Can you work these out from the drawing? Everything is in mm from the part's minimum corner. A direction names the side the tool comes from. Give positions to 0.01 mm unless a question says otherwise; leave off trailing zeros. Order: outer loops, then holes, each group sorted by start corner. A loop starts at its lowest first (then second) coordinate and runs counter-clockwise, first axis right, second up. Notation, with made-up numbers: (-34.5, 58) -> (16.5, 58) arc R23 cw to (16.5, 72) -> close; hole circle Ø9 at (23, -36.75). An arc over 180 degrees is marked (long way). Answer as CSV lines item,"result". Start each with the question number.
(1) I want a section at B-B (z = 32.5). Please give me the cut outline in (x, y), plus the area to 3 significant figures.
(2) I want a section at D-D (y = 16). Please give me the cut outline in (x, z).
(3) I need wall thicknesses on L1, parallel to X at y = 59, z = 6; L2, parallel to X at y = 18, z = 8.5. Which ranges of each line are inside material? Lowest first, please.
(4) I want a section at C-C (y = 73). Please give me the cut outline in (x, z).
(5) Will these pins go through, and if not, where does the flat tip stop? pin 1 Ø8 at (y, z) = (41, 5.5) entering from +X; pin 2 Ø1.5 at (x, y) = (56, 81) entering from +Z; pin 3 Ø5 at (x, z) = (46, 41) entering from +Y; pin 4 Ø3.5 at (x, y) = (59.5, 80) entering from -Z.
(6) On a 3-axis mill with a long thin cutter (end or side, diameter ignored), from which of +Z, -Z, +X, -X, +Y, -Y can I reach the whole of each face in a straight line? I mean the marked faces 1, 2 and 3. Say none if no direction works.
(7) We'd pull the mould along X, two halves only. Please class the marked faces 4, 5 and 6: released by +X, released by -X, zero draft, split by the parting line, or undercut.
(8) I want a section at A-A (x = 42). Please give me the cut outline in (y, z), plus the area to 3 significant figures.
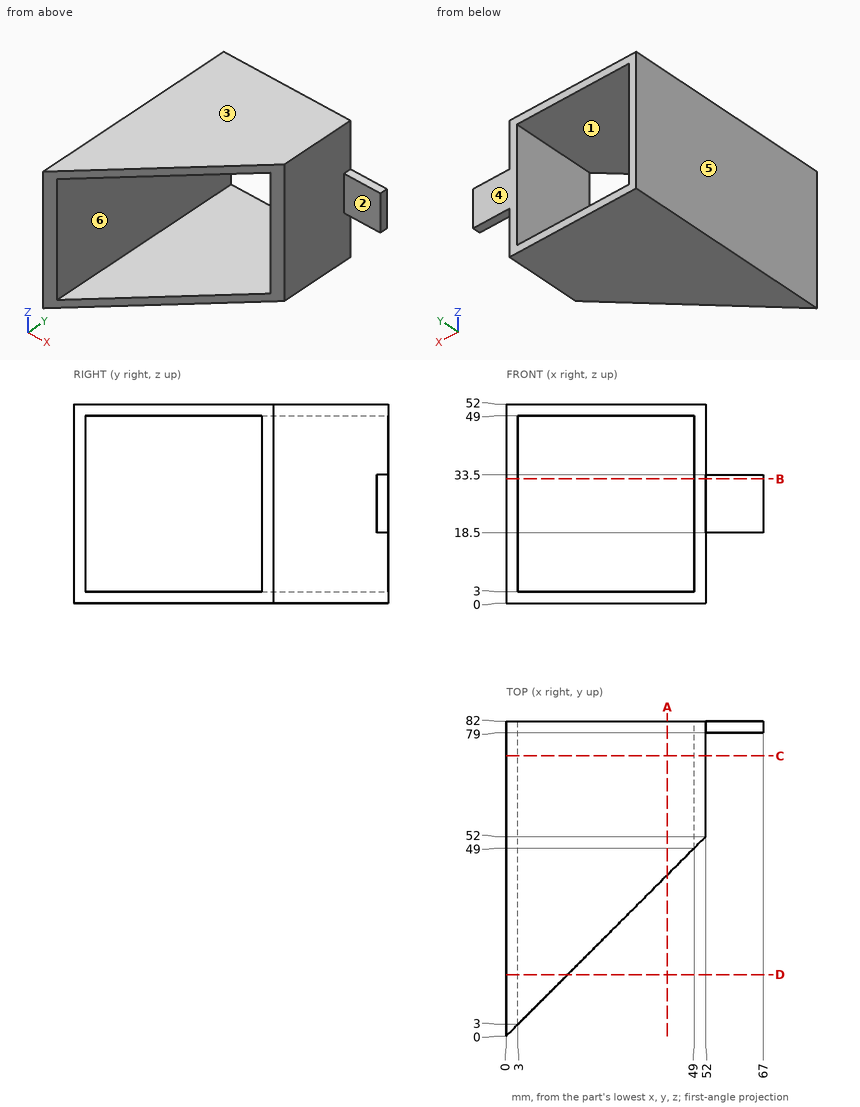
Final values:
1,outline,"(0, 0) -> (3, 3) -> (3, 82) -> (0, 82) -> close; (49, 49) -> (52, 52) -> (52, 79) -> (67, 79) -> (67, 82) -> (49, 82) -> close"
1,area,"381 mm²"
2,outline,"(0, 0) -> (16, 0) -> (16, 3) -> (3, 3) -> (3, 49) -> (16, 49) -> (16, 52) -> (0, 52) -> close"
3,L1,"0 to 3, 49 to 52"
3,L2,"0 to 3"
4,outline,"(0, 0) -> (52, 0) -> (52, 52) -> (0, 52) -> close; hole (3, 3) -> (49, 3) -> (49, 49) -> (3, 49) -> close"
5,pin 1,"x = 44.12"
5,pin 2,"z = 33.5"
5,pin 3,"through"
5,pin 4,"z = 18.5"
6,face 1,"+Y, -Y"
6,face 2,"+Z, -Z, +X, -Y"
6,face 3,"+Z, +X, -X, +Y, -Y"
7,face 4,"zero draft"
7,face 5,"released by -X"
7,face 6,"undercut"
8,outline,"(42, 0) -> (82, 0) -> (82, 3) -> (42, 3) -> close; (42, 49) -> (82, 49) -> (82, 52) -> (42, 52) -> close"
8,area,"240 mm²"
